Autodesk Inventor part; units mm, degrees
ref_plane "YZ Plane" through (0, 0, 0) normal (1, 0, 0) x (0, 1, 0)
ref_plane "XZ Plane" through (0, 0, 0) normal (0, 1, 0) x (-1, 0, 0)
ref_plane "XY Plane" through (0, 0, 0) normal (0, 0, 1) x (1, 0, 0)
sketch "Sketch1" plane through (0, 0, 0) normal (0, 0, 1) x (1, 0, 0)
  line L0 (0, 0) -> (50.8, 0)
  line L1 (50.8, 0) -> (50.8, 50.8)
  line L2 (50.8, 50.8) -> (0, 50.8)
  line L3 (0, 50.8) -> (0, 0)
  dimension "d0" = 50.8
  dimension "d1" = 50.8
extrude "Extrusion1" add sketch "Sketch1" along normal blind 101.6
sketch "Sketch2" plane through (0, 0, 101.6) normal (0, 0, 1) x (1, 0, 0)
  line L0 (50.8, 50.8) -> (0, 50.8)
  line L1 (25.4, 38.1) -> (12.7, 38.1)
  line L2 (12.7, 38.1) -> (38.1, 38.1)
  line L3 (38.1, 38.1) -> (38.1, 12.7)
  line L4 (38.1, 12.7) -> (12.7, 12.7)
  line L5 (12.7, 12.7) -> (12.7, 38.1)
  point P0 (0, 0)
  dimension "d8" = 25.4
  dimension "d9" = 25.4
extrude "Extrusion2" add sketch "Sketch2" along normal blind 31.75
sketch "Sketch3" plane through (0, 50.8, 0) normal (0, 1, 0) x (1, 0, 0)
  line L0 (50.8, 0) -> (0, 0)
  line L1 (25.4, 0) -> (25.4, -25.4)
  line L2 (25.4, -25.4) -> (19.05, -25.4)
  line L3 (19.05, -25.4) -> (19.05, -12.7)
  line L4 (19.05, -12.7) -> (25.4, -12.7)
  line L5 (25.4, -12.7) -> (25.4, -25.4)
  line L6 (25.4, -25.4) -> (31.75, -25.4)
  line L7 (31.75, -25.4) -> (31.75, -12.7)
  line L8 (31.75, -12.7) -> (25.4, -12.7)
  line L9 (25.4, -12.7) -> (25.4, -25.4)
  dimension "d12" = 25.4
  dimension "d13" = 6.35
  dimension "d14" = 12.7
  dimension "d15" = 6.35
extrude "Extrusion3" cut sketch "Sketch3" against normal blind 25.4
sketch "Sketch4" plane through (0, 50.8, 0) normal (0, 1, 0) x (1, 0, 0)
  line L0 (19.05, -25.4) -> (19.05, -12.7)
  line L1 (19.05, -19.05) -> (15.875, -19.05)
  line L2 (0, 0) -> (0, -101.6)
  line L3 (15.875, -19.05) -> (34.925, -19.05)
  line L4 (34.925, -19.05) -> (34.925, -28.575)
  line L5 (34.925, -28.575) -> (15.875, -28.575)
  line L6 (15.875, -28.575) -> (15.875, -19.05)
  line L7 (34.925, -19.05) -> (15.875, -19.05)
  line L8 (15.875, -19.05) -> (15.875, -9.525)
  line L9 (15.875, -9.525) -> (34.925, -9.525)
  line L10 (34.925, -9.525) -> (34.925, -19.05)
  dimension "d18" = 3.175
  dimension "d19" = 19.05
  dimension "d20" = 9.525
  dimension "d21" = 19.05
  dimension "d22" = 9.525
extrude "Extrusion4" cut sketch "Sketch4" against normal blind 25.4
properties part number "SquareCrank_SBail"
Source: CAD feature listing. Evaluate the final solid. Frame: model axes, mm. A direction names the side the tool comes from. Round coordinates to 2 decimals unless told otherwise and drop trailing zeros. Loops run counter-clockwise (first coordinate to the right, second up) from the corner with the lowest first, then second, coordinate; pieces in that order, holes last.
Q1. Section B-B, the plane z = 25. Return loops of the section in (x, y) (3 decimals), plus the area to 3 significant figures.
Q2. First-contact query: P1, Ø5, axis at y = 22, z = 118.5, coming from the +X side; P2, Ø12.5, axis at x = 29, z = 114.5, coming from the -Y side; P3, Ø20.5, axis at y = 25, z = 123, coming from the -X side. Flat tips, straight axial feed; report the tip coordinate or a pass-through.
Q3. Ray query, line 1 (X direction, y = 40, z = 11.5) (3 decimals); line 2 (Z direction, x = 25, y = 28) (3 decimals); line 3 (X direction, y = 19.5, z = 114). Return the intervals inside material, ascending.
Q4. Access query for faces 1 (the face through (26, 12.7, 117)), 2 (the face through (25, 25.4, 19)), 3 (the face through (38.1, 26, 117)), 4 (the face through (12.7, 25, 117)), 5 (the face through (26, 38.1, 117)). Directions: +Z, -Z, +X, -X, +Y, -Y. A direction counts if a zero-diameter tool reaches every point of the face in a straight line with its end or side. Return the directions, or none.
Q5. Section C-C, the plane x = 21. Return loops of the section in (y, z) (3 decimals).
Q6. Mould query, pull axis Z, two halves, no side actions, for faces 6 (the face through (25, 26, 133.35)), 7 (the face through (25, 38, 9.525)), 8 (the face through (25, 0, 50)), 9 (the face through (34.925, 38, 19)). Classes: pulls with the +Z half, pulls with the -Z half, needs draft (parallel to the pull), parting line crosses it, or undercut.
Q7. Section D-D, the plane y = 22.5. Return loops of the section in (x, z), plus the area to 3 significant figures.
Q8. Section A-A, the plane y = 29. Return loops of the section in (x, z) (3 decimals).
Solutions:
1. outline: (0, 0) - (50.8, 0) - (50.8, 50.8) - (34.925, 50.8) - (34.925, 25.4) - (15.875, 25.4) - (15.875, 50.8) - (0, 50.8) - close
1. area: 2,100 mm2
2. P1: stops at x = 38.1
2. P2: stops at y = 12.7
2. P3: stops at x = 12.7
3. line 1: x = 0 to 15.875, 34.925 to 50.8
3. line 2: z = 0 to 9.525, 28.575 to 133.35
3. line 3: x = 12.7 to 38.1
4. face 1: +Z, +X, -X, -Y
4. face 2: +Y
4. face 3: +Z, +X, +Y, -Y
4. face 4: +Z, -X, +Y, -Y
4. face 5: +Z, +X, -X, +Y
5. outline: (0, 0) - (50.8, 0) - (50.8, 9.525) - (25.4, 9.525) - (25.4, 28.575) - (50.8, 28.575) - (50.8, 101.6) - (38.1, 101.6) - (38.1, 133.35) - (12.7, 133.35) - (12.7, 101.6) - (0, 101.6) - close
6. face 6: pulls with the +Z half
6. face 7: undercut
6. face 8: needs draft
6. face 9: undercut
7. outline: (0, 0) - (50.8, 0) - (50.8, 101.6) - (38.1, 101.6) - (38.1, 133.35) - (12.7, 133.35) - (12.7, 101.6) - (0, 101.6) - close
7. area: 5,970 mm2
8. outline: (0, 0) - (50.8, 0) - (50.8, 101.6) - (38.1, 101.6) - (38.1, 133.35) - (12.7, 133.35) - (12.7, 101.6) - (0, 101.6) - close; hole (15.875, 9.525) - (34.925, 9.525) - (34.925, 28.575) - (15.875, 28.575) - close
